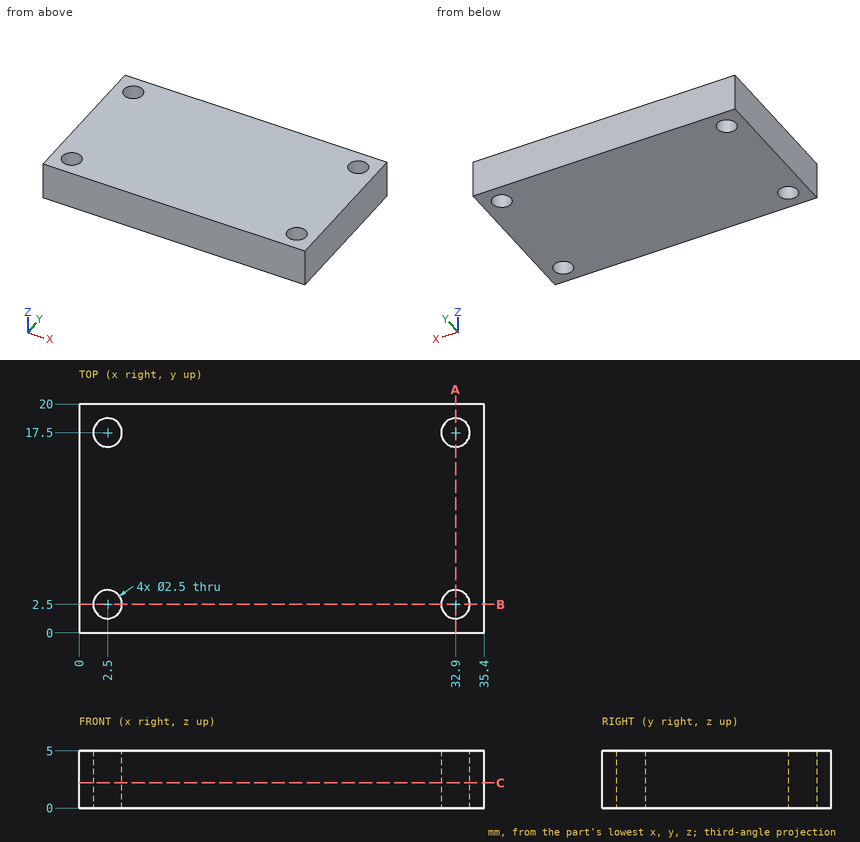
Here's the drawing with two shaded views (mm, measured from the low corner). I have some questions. Give positions to 0.01 mm unless a question says otherwise; leave off trailing zeros. Write each loop counter-clockwise with the first axis right and the second up, starting at its lowest first coordinate (ties: lowest second). Pieces come first, ordered by that corner, then holes. Notation, with made-up numbers: (-3.75, 43) -> (25.25, 43) arc R27 ccw to (25.25, 82) -> close; hole circle Ø2 at (7.25, -26.5). An arc over 180 degrees is marked (long way). Use one line per item in the form item = value. Start each with the question number.
1. Imagine slicing it at C-C on z = 2.2. List the corners of the cut face in (x, y) for me.
2. Imagine slicing it at B-B on y = 2.5. List the corners of the cut face in (x, z) for me.
3. If I drill on L1, parallel to Y at x = 33, z = 3.5; L2, parallel to X at y = 1.5, z = 3.15; L3, parallel to X at y = 17, z = 3, over which ranges is the centre line in solid material (lowest first)?
4. Imagine slicing it at A-A on x = 32.9. List the corners of the cut face in (y, z) for me.
Entries:
q1.outline = (0, 0) -> (35.4, 0) -> (35.4, 20) -> (0, 20) -> close; hole circle Ø2.5 at (2.5, 2.5); hole circle Ø2.5 at (2.5, 17.5); hole circle Ø2.5 at (32.9, 2.5); hole circle Ø2.5 at (32.9, 17.5)
q2.outline = (0, 0) -> (1.25, 0) -> (1.25, 5) -> (0, 5) -> close; (3.75, 0) -> (31.65, 0) -> (31.65, 5) -> (3.75, 5) -> close; (34.15, 0) -> (35.4, 0) -> (35.4, 5) -> (34.15, 5) -> close
q3.L1 = 0 to 1.25, 3.75 to 16.25, 18.75 to 20
q3.L2 = 0 to 1.75, 3.25 to 32.15, 33.65 to 35.4
q3.L3 = 0 to 1.35, 3.65 to 31.75, 34.05 to 35.4
q4.outline = (0, 0) -> (1.25, 0) -> (1.25, 5) -> (0, 5) -> close; (3.75, 0) -> (16.25, 0) -> (16.25, 5) -> (3.75, 5) -> close; (18.75, 0) -> (20, 0) -> (20, 5) -> (18.75, 5) -> close
